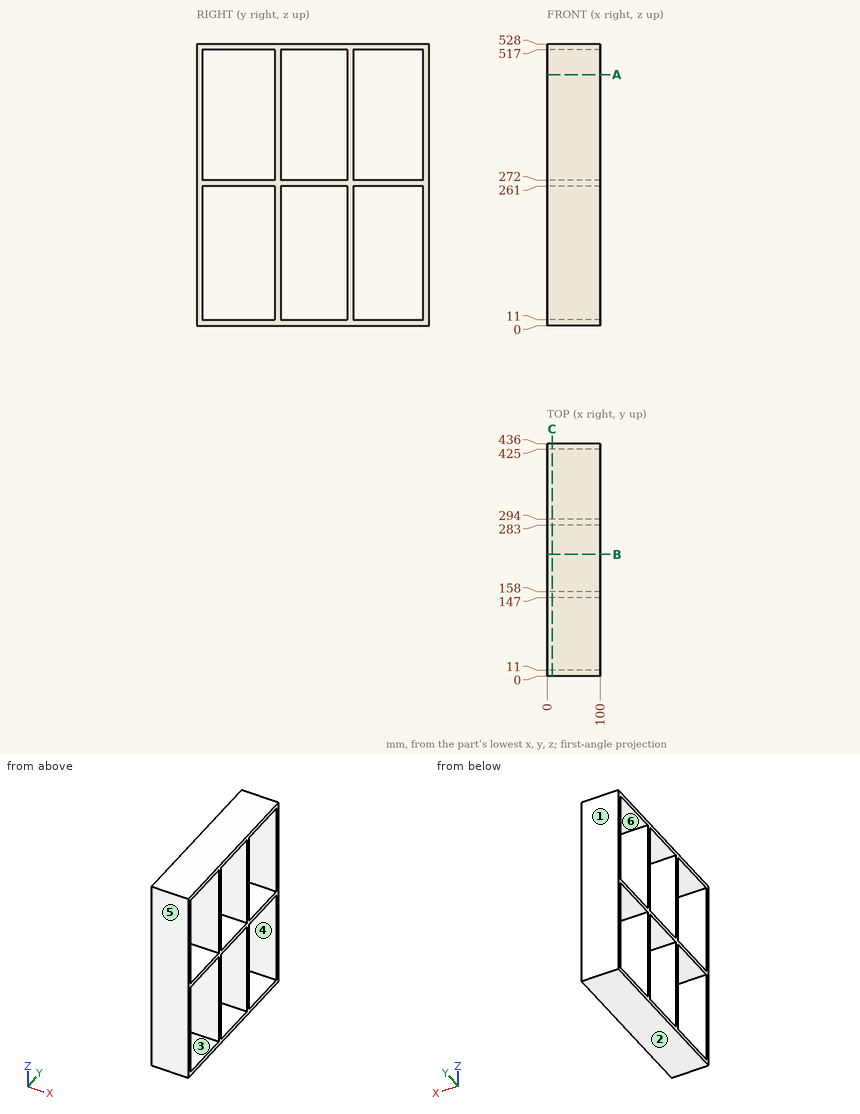
Drawing for the job (mm, zero at the part's lowest x, y, z). A direction names the side the tool comes from. Coordinates: 2 decimals unless noted, no trailing zeros. Order: outer loops, then holes, each group sorted by start corner. A loop starts at its lowest first (then second) coordinate and runs counter-clockwise, first axis right, second up. Notation, with made-up numbers: (54.25, 24.5) -> (76.25, 24.5) arc R17 cw to (76.25, 51.5) -> close; hole circle Ø8 at (-38, -30). An arc over 180 degrees is marked (long way). Answer in a Markdown table with one row per item.
1) Band-saw the part on A-A (z = 470.5). List the corners of the cut face in (x, y).
Check values:
| item | result |
|---|---|
| outline | (0, 0) -> (100, 0) -> (100, 11) -> (0, 11) -> close; (0, 147) -> (100, 147) -> (100, 158) -> (0, 158) -> close; (0, 283) -> (100, 283) -> (100, 294) -> (0, 294) -> close; (0, 425) -> (100, 425) -> (100, 436) -> (0, 436) -> close |
2) Band-saw the part on C-C (x = 9.5). List the corners of the cut face in (y, z), and give its area (3 significant figures).
Check values:
| item | result |
|---|---|
| outline | (0, 0) -> (436, 0) -> (436, 528) -> (0, 528) -> close; hole (11, 11) -> (147, 11) -> (147, 261) -> (11, 261) -> close; hole (11, 272) -> (147, 272) -> (147, 517) -> (11, 517) -> close; hole (158, 11) -> (283, 11) -> (283, 261) -> (158, 261) -> close; hole (158, 272) -> (283, 272) -> (283, 517) -> (158, 517) -> close; hole (294, 11) -> (425, 11) -> (425, 261) -> (294, 261) -> close; hole (294, 272) -> (425, 272) -> (425, 517) -> (294, 517) -> close |
| area | 36,200 mm2 |
3) Which spindle directions (+Z, -Z, +X, -X, +Y, -Y) get a long thin tool onto all of the face, cutting with end or side? Do the marked faces 5 and 6. Say none if no direction does.
Check values:
| item | result |
|---|---|
| face 5 | +Z, -Z, +X, -X, -Y |
| face 6 | +X, -X |
4) Band-saw the part on B-B (y = 228). List the corners of the cut face in (x, z).
Check values:
| item | result |
|---|---|
| outline | (0, 0) -> (100, 0) -> (100, 11) -> (0, 11) -> close; (0, 261) -> (100, 261) -> (100, 272) -> (0, 272) -> close; (0, 517) -> (100, 517) -> (100, 528) -> (0, 528) -> close |
5) Flat gauge pin, fed straight in: P1, Ø5, axis at x = 82.5, z = 175, coming from the -Y side. Where does the tip first touch, or does it go through?
Check values:
| item | result |
|---|---|
| P1 | y = 0 |
6) Drill centre lines: line 1 (Y direction, x = 26.5, z = 287.5); line 2 (Z direction, x = 31.5, y = 222). Where is each one in solid material? Low to high.
Check values:
| item | result |
|---|---|
| line 1 | 0 to 11, 147 to 158, 283 to 294, 425 to 436 |
| line 2 | 0 to 11, 261 to 272, 517 to 528 |
7) Mould opens along Z. For the marked faces 1, 2, 3 and 4 say: pulls with the +Z half, pulls with the -Z half, needs draft (parallel to the pull), parting line crosses it, or undercut.
Check values:
| item | result |
|---|---|
| face 1 | needs draft |
| face 2 | pulls with the -Z half |
| face 3 | undercut |
| face 4 | undercut |
